Geometry: final body of the model. Coordinates: model frame, mm. A direction names the side the tool comes from. Coordinates: 2 decimals unless noted, no trailing zeros. Write each loop counter-clockwise with the first axis right and the second up, starting at its lowest first coordinate (ties: lowest second). Pieces come first, ordered by that corner, then holes.
from build123d import *

# Parameters (mm, degrees)
SKETCH1_R               = 9.1313
BOSS_EXTRUDE1_DEPTH     = 41.783
CUT_EXTRUDE1_DEPTH      = 44.733058073
CUT_EXTRUDE1_DEPTH_BACK = 44.733058073
SKETCH2_R               = 3.3782
CUT_EXTRUDE3_DEPTH      = 44.73305821
CUT_EXTRUDE3_DEPTH_BACK = 44.73305821
SKETCH3_W               = 10.5156
SKETCH3_H               = 6.1214


with BuildPart() as part:
    # Sketch1 → Boss-Extrude1 (new body)
    with BuildSketch(Plane.XY):
        Circle(SKETCH1_R)
    extrude(amount=BOSS_EXTRUDE1_DEPTH)

    # Sketch2 → Cut-Extrude1 (cut, two sides: drawn at the far end of the back side and taken through both)
    with BuildSketch(Plane(origin=(0, 0, 0), x_dir=(0, 0, -1), z_dir=(1, 0, 0)).offset(-CUT_EXTRUDE1_DEPTH_BACK)):
        with Locations((-21.9202, 0)):
            Circle(SKETCH2_R)
    extrude(amount=CUT_EXTRUDE1_DEPTH + CUT_EXTRUDE1_DEPTH_BACK, mode=Mode.SUBTRACT)

    # Sketch3 → Cut-Extrude3 (cut, two sides: drawn at the far end of the back side and taken through both)
    with BuildSketch(Plane(origin=(0, 0, 0), x_dir=(0, 0, -1), z_dir=(1, 0, 0)).offset(-CUT_EXTRUDE3_DEPTH_BACK)):
        with Locations((-36.5252, 0)):
            Rectangle(SKETCH3_W, SKETCH3_H)
    extrude(amount=CUT_EXTRUDE3_DEPTH + CUT_EXTRUDE3_DEPTH_BACK, mode=Mode.SUBTRACT)


solid = part.part
Item 1: Section D-D, the plane x = -4. Output: boundary loops of the cut face in (y, z), plus the area to 3 significant figures.
Derived:
outline: (-8.21, 0) - (8.21, 0) - (8.21, 41.78) - (3.06, 41.78) - (3.06, 31.27) - (-3.06, 31.27) - (-3.06, 41.78) - (-8.21, 41.78) - close; hole circle Ø6.76 at (0, 21.92)
area: 586 mm2
Item 2: Pull-direction query (Y, two-part tool) for faces 1 (the cylindrical face through (4.214, -8.101, 20.599)), 2 (the flat face through (0, -5, 41.783)), 3 (the cylindrical face through (-0.1, -1.3, 18.8)); classes: released by +Y, released by -Y, zero draft, split by the parting line, or undercut.
Derived:
face 1: split by the parting line
face 2: zero draft
face 3: undercut
Item 3: Section C-C, the plane x = 0. Output: boundary loops of the cut face in (y, z), plus the area to 3 significant figures.
Derived:
outline: (-9.13, 0) - (9.13, 0) - (9.13, 41.78) - (3.06, 41.78) - (3.06, 31.27) - (-3.06, 31.27) - (-3.06, 41.78) - (-9.13, 41.78) - close; hole circle Ø6.76 at (0, 21.92)
area: 663 mm2
Item 4: Material intervals for probe 1 along Z at (x, y) = (0.5, 0); probe 2 along Y at (x, z) = (1.5, 37); probe 3 along Z at (x, y) = (-0.25, 2.25), sorted ascending.
Derived:
probe 1: z = 0 to 18.54, 25.3 to 31.27
probe 2: y = -9.01 to -3.06, 3.06 to 9.01
probe 3: z = 0 to 19.4, 24.44 to 31.27
Item 5: Pin query (flat end, axial travel): pin 1 (1.5 mm diameter, centred on x = -2.5, z = 15.5, fed in from +Y); pin 2 (4 mm diameter, centred on x = 5, z = 9.5, fed in from -Y); pin 3 (2 mm diameter, centred on y = 4, z = 20, fed in from +X); pin 4 (5.5 mm diameter, centred on y = 0, z = 21.92, fed in from -X). Return the tip coordinate at first contact, or that it passes through.
Derived:
pin 1: stops at y = 8.96
pin 2: stops at y = -8.62
pin 3: stops at x = 8.62
pin 4: passes through
Item 6: Section B-B, the plane z = 39. Output: boundary loops of the cut face in (x, y), plus the area to 3 significant figures.
Derived:
outline: (-8.6, -3.06) arc R9.13 ccw to (8.6, -3.06) - close; (-8.6, 3.06) - (8.6, 3.06) arc R9.13 ccw to start
area: 152 mm2
Item 7: Set-up query: faces 4 (the flat face through (0, 5, 41.783)), 5 (the flat face through (0, 3.061, 37)). Return all of +Z, -Z, +X, -X, +Y, -Y with unobstructed straight access to the full face (end or side cutting, diameter ignored); none if empty.
Derived:
face 4: +Z, +X, -X, +Y, -Y
face 5: +Z, +X, -X
Item 8: Section A-A, the plane y = 0. Output: boundary loops of the cut face in (x, z).
Derived:
outline: (-9.13, 0) - (9.13, 0) - (9.13, 18.54) - (-9.13, 18.54) - close; (-9.13, 25.3) - (9.13, 25.3) - (9.13, 31.27) - (-9.13, 31.27) - close
